Build history of the part. All positions in model axes, mm. Face numbers are marked on the shaded views. A direction names the side the tool comes from. Coordinates: 2 decimals unless noted, no trailing zeros. Loops run counter-clockwise (first coordinate to the right, second up) from the corner with the lowest first, then second, coordinate; pieces in that order, holes last.
(1) Two-plate mould, pull along X, no slides. Class the marked faces 1, 2, 3 and 4: pulls with the +X half, pulls with the -X half, needs draft (parallel to the pull), parting line crosses it, or undercut.
(2) Flat gauge pins, fed straight in: P1, Ø6, axis at x = 10, z = 6, coming from the -Y side; P2, Ø4, axis at y = -13.5, z = 3.5, coming from the +X side; P3, Ø2, axis at x = -11, z = 9.5, coming from the -Y side. Where does each tip first touch, or does it go through?
(3) Slice it at A-A (x = 0). Give the cut face in (y, z) (1 decimal), and give its area (3 significant figures).
(4) Slice it at C-C (z = 2). Give the cut face in (x, y) (1 decimal).
(5) Tool access for the marked faces 5, 6, 7, 8 and 9: list every direction of +Z, -Z, +X, -X, +Y, -Y with a clear straight run to the whole face (end or side of a thin tool).
(6) Wall check: L1, parallel to Y at x = 0, z = 4.75 (3 decimals); L2, parallel to Y at x = 14.5, z = 8.25; L3, parallel to X at y = -15, z = 9.75. Give the ranges that are in metal, low to high.
(7) Slice it at B-B (z = 6). Give the cut face in (x, y) (1 decimal).
from build123d import *

# Parameters (mm, degrees)
BOSS_EXTRUDE1_DEPTH                           = 10.668
CSK_FOR_2_FLAT_HEAD_MACHINE_SCREW1_AT_2_COUNT = 2
CSK_FOR_2_FLAT_HEAD_MACHINE_SCREW1_AT_2_PITCH = 28.241625
CSK_FOR_2_FLAT_HEAD_MACHINE_SCREW1_AT_3_COUNT = 2
CSK_FOR_2_FLAT_HEAD_MACHINE_SCREW1_AT_3_PITCH = 24.379834317
SKETCH4_R                                     = 6.477
CUT_EXTRUDE1_DEPTH                            = 1.5748
SKETCH5_R                                     = 4.7879
CUT_EXTRUDE2_DEPTH                            = 11.668
SKETCH6_W                                     = 8.0264
SKETCH6_H                                     = 10.033
CUT_EXTRUDE3_DEPTH                            = 5.08
DRAFT2_ANGLE                                  = 45
CHAMFER1_SIZE                                 = 3.175
CHAMFER2_SIZE                                 = 6.35
CUT_EXTRUDE4_DEPTH                            = 2.7432


with BuildPart() as part:
    # Sketch1 → Boss-Extrude1 (new body)
    with BuildSketch(Plane.XY):
        Polygon((21.463, 7.1882), (-18.288, 7.1882), (-18.288, -7.1882), (-7.1882, -7.1882), (-7.1882, -23.495), (7.1882, -23.495), (7.1882, -7.1882), (21.463, -7.1882), align=None)
    extrude(amount=BOSS_EXTRUDE1_DEPTH)

    # Sketch3 → CSK for #2 Flat Head Machine Screw1 (revolve, cut)
    with BuildSketch(Plane(origin=(15.859125, 0, 10.668), x_dir=(0, -1, 0), z_dir=(1, 0, 0))):
        Polygon((0, 0), (0, 10.668), (1.2192, 10.668), (1.2192, 3.853535587), (2.1844, 2.7432), (2.1844, 0), align=None)
    csk_for_2_flat_head_machine_screw1 = revolve(axis=Axis((15.859125, 0, 17.018), (0, 0, -1)), mode=Mode.SUBTRACT)

    # CSK for #2 Flat Head Machine Screw1 at 2: CSK for #2 Flat Head Machine Screw1 ×2
    with Locations(*[(-i * CSK_FOR_2_FLAT_HEAD_MACHINE_SCREW1_AT_2_PITCH, 0, 0) for i in range(1, CSK_FOR_2_FLAT_HEAD_MACHINE_SCREW1_AT_2_COUNT)]):
        add(csk_for_2_flat_head_machine_screw1, mode=Mode.SUBTRACT)

    # CSK for #2 Flat Head Machine Screw1 at 3: CSK for #2 Flat Head Machine Screw1 ×2
    with Locations(*[Vector(-0.650501755, -0.759504751, 0) * (i * CSK_FOR_2_FLAT_HEAD_MACHINE_SCREW1_AT_3_PITCH) for i in range(1, CSK_FOR_2_FLAT_HEAD_MACHINE_SCREW1_AT_3_COUNT)]):
        add(csk_for_2_flat_head_machine_screw1, mode=Mode.SUBTRACT)

    # Sketch4 → Cut-Extrude1 (cut)
    with BuildSketch(Plane.XY.offset(10.668)):
        Circle(SKETCH4_R)
    extrude(amount=-CUT_EXTRUDE1_DEPTH, mode=Mode.SUBTRACT)

    # Sketch5 → Cut-Extrude2 (cut, through all)
    with BuildSketch(Plane.XY.offset(10.668)):
        Circle(SKETCH5_R)
    extrude(amount=-CUT_EXTRUDE2_DEPTH, mode=Mode.SUBTRACT)

    # Sketch6 → Cut-Extrude3 (cut)
    with BuildSketch(Plane(origin=(0, 0, 0), x_dir=(-1, 0, 0), z_dir=(0, 0, -1))):
        with Locations((-6.24205, 10.483214746)):
            Rectangle(SKETCH6_W, SKETCH6_H)
    extrude(amount=-CUT_EXTRUDE3_DEPTH, mode=Mode.SUBTRACT)

    # Draft2
    draft2_faces = [part.faces().sort_by_distance(p)[0] for p in [
        (6.24205, 6.327457373, 5.08),
    ]]
    draft(draft2_faces, Plane(origin=(10.25525, 5.466714746, 5.08), x_dir=(1, 0, 0), z_dir=(0, 1, 0)), DRAFT2_ANGLE)

    # Chamfer1
    chamfer1_edges = [part.edges().sort_by_distance(p)[0] for p in [
        (21.463, -7.1882, 5.334),
        (7.1882, -23.495, 5.334),
        (-7.1882, -23.495, 5.334),
        (-18.288, -7.1882, 5.334),
        (-18.288, 7.1882, 5.334),
        (21.463, 7.1882, 5.334),
    ]]
    chamfer(chamfer1_edges, length=CHAMFER1_SIZE)

    # Chamfer2
    chamfer2_edges = [part.edges().sort_by_distance(p)[0] for p in [
        (7.1882, -7.1882, 5.334),
        (-7.1882, -7.1882, 5.334),
    ]]
    chamfer(chamfer2_edges, length=CHAMFER2_SIZE)

    # Sketch7 → Cut-Extrude4 (cut)
    with BuildSketch(Plane.XY.offset(10.668)):
        with BuildLine():
            Line((3.7719, -14.70943597), (7.183135951, -11.298200019))
            Line((7.183135951, -11.298200019), (3.260798724, -7.375862792))
            ThreePointArc((3.260798724, -7.375862792), (0, -8.0645), (-3.260798724, -7.375862792))
            Line((-3.260798724, -7.375862792), (-7.183135951, -11.298200019))
            Line((-7.183135951, -11.298200019), (-3.7719, -14.70943597))
            Line((-3.7719, -14.70943597), (-3.7719, -18.5166))
            ThreePointArc((-3.7719, -18.5166), (0, -22.2885), (3.7719, -18.5166))
            Line((3.7719, -18.5166), (3.7719, -14.70943597))
        make_face()
        with BuildLine():
            Line((12.88063597, -5.6007), (17.63043597, -5.6007))
            Line((17.63043597, -5.6007), (19.8755, -3.35563597))
            Line((19.8755, -3.35563597), (19.8755, 3.35563597))
            Line((19.8755, 3.35563597), (17.63043597, 5.6007))
            Line((17.63043597, 5.6007), (8.0645, 5.6007))
            Line((8.0645, 5.6007), (8.0645, 0))
            ThreePointArc((8.0645, 0), (7.500371575, -2.963205441), (5.886910197, -5.511846205))
            Line((5.886910197, -5.511846205), (9.428199981, -9.053135989))
            Line((9.428199981, -9.053135989), (12.88063597, -5.6007))
        make_face()
        with BuildLine():
            Line((-14.45543597, 5.6007), (-16.7005, 3.35563597))
            Line((-16.7005, 3.35563597), (-16.7005, -3.35563597))
            Line((-16.7005, -3.35563597), (-14.45543597, -5.6007))
            Line((-14.45543597, -5.6007), (-12.88063597, -5.6007))
            Line((-12.88063597, -5.6007), (-9.428199981, -9.053135989))
            Line((-9.428199981, -9.053135989), (-5.886910197, -5.511846205))
            ThreePointArc((-5.886910197, -5.511846205), (-7.500371575, -2.963205441), (-8.0645, 0))
            Line((-8.0645, 0), (-8.0645, 5.6007))
            Line((-8.0645, 5.6007), (-14.45543597, 5.6007))
        make_face()
    extrude(amount=-CUT_EXTRUDE4_DEPTH, mode=Mode.SUBTRACT)


solid = part.part
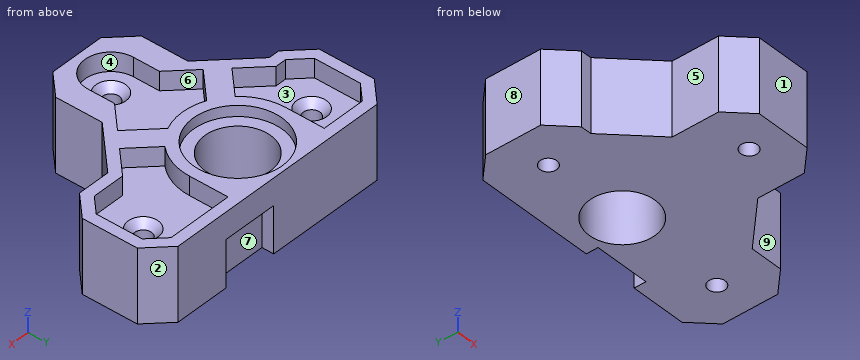
Response values:
1. face 1: needs draft
1. face 2: pulls with the +X half
1. face 3: undercut
1. face 4: undercut
2. P1: stops at y = -20.51
2. P2: stops at x = 9.23
2. P3: stops at y = -10.73
3. outline: (-23.5, 0) - (-19.7, 0) - (-19.7, 6.8) - (-20.7, 7.9) - (-22.3, 7.9) - (-22.3, 10.7) - (-23.5, 10.7) - close; (-17.3, 0) - (-4.8, 0) - (-4.8, 9.1) - (-6.5, 9.1) - (-6.5, 10.7) - (-8.1, 10.7) - (-8.1, 7.9) - (-16.3, 7.9) - (-17.3, 6.8) - close; (4.8, 0) - (7.2, 0) - (7.2, 10.7) - (6.5, 10.7) - (6.5, 9.1) - (4.8, 9.1) - close
3. area: 160 mm2
4. outline: (-18.3, -4) - (-15.1, -7.2) - (-13.5, -7.2) - (-7.2, -13.5) - (-7.2, -20.3) - (-4, -23.5) - (4, -23.5) - (7.2, -20.3) - (7.2, -13.5) - (13.5, -7.2) - (18.3, -7.2) - (21.5, -4) - (21.5, 4) - (18.3, 7.2) - (10.3, 7.2) - (10.3, 5.5) - (2.2, 5.5) - (2.2, 7.2) - (-15.1, 7.2) - (-18.3, 4) - close; hole circle Ø2.4 at (-12.4, 0); hole circle Ø9.6 at (0, 0); hole circle Ø2.4 at (0, -18.5); hole circle Ø2.4 at (15.9, 0)
5. face 5: +Z, -Z, -X, -Y
5. face 6: +Z
5. face 7: -Z, +Y
5. face 8: +Z, -Z, -X, +Y, -Y
5. face 9: +Z, -Z, +X, -Y
6. L1: y = -23.495 to -19.736, -17.297 to -4.788, 4.788 to 7.188
6. L2: y = -7.19 to -5.6, 5.6 to 7.19
6. L3: x = -7.19 to -3.77, 3.77 to 7.19
7. outline: (-18.3, -4) - (-15.1, -7.2) - (-13.5, -7.2) - (-7.2, -13.5) - (-7.2, -20.3) - (-4, -23.5) - (4, -23.5) - (7.2, -20.3) - (7.2, -13.5) - (13.5, -7.2) - (18.3, -7.2) - (21.5, -4) - (21.5, 4) - (18.3, 7.2) - (10.3, 7.2) - (10.3, 6.4) - (2.2, 6.4) - (2.2, 7.2) - (-15.1, 7.2) - (-18.3, 4) - close; hole circle Ø2.4 at (-12.4, 0); hole circle Ø9.6 at (0, 0); hole circle Ø2.4 at (0, -18.5); hole circle Ø2.4 at (15.9, 0)
